```python
from build123d import *

# Parameters (mm, degrees)
F1_DEPTH = 190


# Not quite as in the source:
# - a feature names something its author has since deleted; it is built from what else it names


with BuildPart() as f1:
    # F0 (on Front) → F1 (new body)
    with BuildSketch(Plane.XZ):
        with BuildLine():
            Line((-32.5, -80), (32.5, -80))
            Line((32.5, -80), (32.5, -69.5))
            Line((32.5, -69.5), (-19, -69.5))
            ThreePointArc((-19, -69.5), (-23.2426406871, -67.7426406871), (-25, -63.5))
            Line((-25, -63.5), (-25, 18))
            Line((-25, 18), (-32.5, 18))
            Line((-32.5, 18), (-32.5, -80))
        make_face()
    extrude(amount=-F1_DEPTH)


solid = f1.part
```
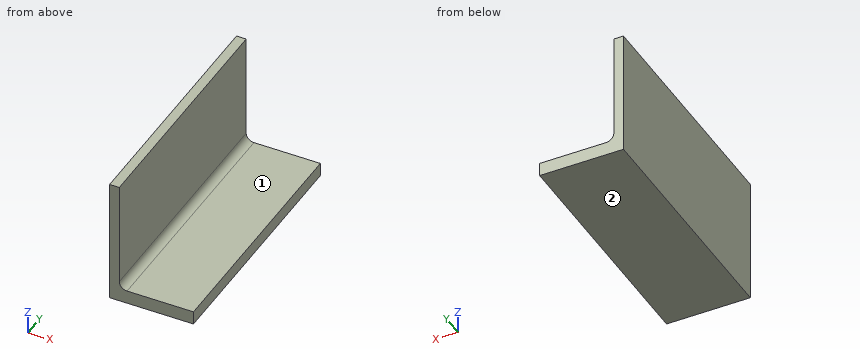
Geometry: final body of the model. Coordinates: model frame, mm. Face numbers are marked on the shaded views. A direction names the side the tool comes from. Round coordinates to 2 decimals unless told otherwise and drop trailing zeros. Write each loop counter-clockwise with the first axis right and the second up, starting at its lowest first coordinate (ties: lowest second). Pieces come first, ordered by that corner, then holes.
Item 1: Material intervals for L1, parallel to X at y = 26, z = -16.5; L2, parallel to Z at x = -13, y = 67; L3, parallel to Z at x = -21, y = 63, sorted ascending.
Item 2: Section query A-A (y = 35.5). Return loops of the section in (x, z), plus the area to 3 significant figures.
Item 3: Set-up query: the marked faces 1 and 2. Return all of +Z, -Z, +X, -X, +Y, -Y with unobstructed straight access to the full face (end or side cutting, diameter ignored); none if empty.
Item 4: Section query C-C (z = 6). Return loops of the section in (x, y), plus the area to 4 significant figures.
Item 5: Section query B-B (x = 25). Return loops of the section in (y, z), plus the area to 4 significant figures.
Item 6: Pin query (flat end, axial travel): P1, Ø24.5, axis at y = 102.5, z = -32.5, coming from the +X side; P2, Ø1.5, axis at x = -9.5, y = 48, coming from the +Z side; P3, Ø1.5, axis at x = -22, y = 164, coming from the +Z side. Return the tip coordinate at first contact, or that it passes through.
Completed:
1. L1: x = -32.5 to -25
1. L2: z = -80 to -69.5
1. L3: z = -80 to -69.16
2. outline: (-32.5, -80) - (32.5, -80) - (32.5, -69.5) - (-19, -69.5) arc R6 cw to (-25, -63.5) - (-25, 18) - (-32.5, 18) - close
2. area: 1,350 mm2
3. face 1: +Z, +X, +Y, -Y
3. face 2: -Z, +X, -X, +Y, -Y
4. outline: (-32.5, 0) - (-25, 0) - (-25, 190) - (-32.5, 190) - close
4. area: 1,425 mm2
5. outline: (0, -80) - (190, -80) - (190, -69.5) - (0, -69.5) - close
5. area: 1,995 mm2
6. P1: stops at x = -25
6. P2: stops at z = -69.5
6. P3: stops at z = -68.18
